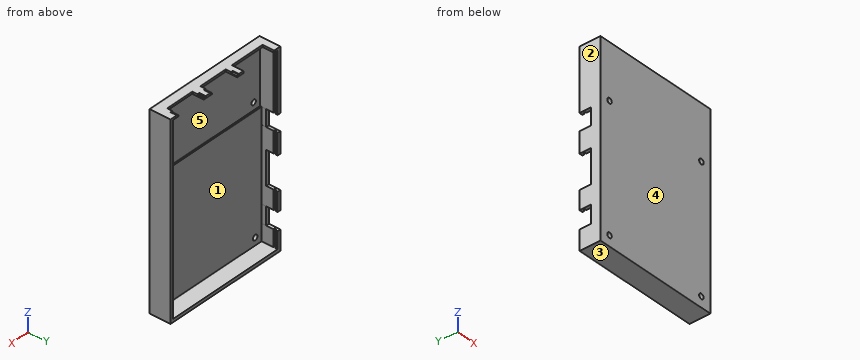
Autodesk Inventor part; units mm, degrees
ref_plane "YZ Plane" through (0, 0, 0) normal (1, 0, 0) x (0, 1, 0)
ref_plane "XZ Plane" through (0, 0, 0) normal (0, 1, 0) x (-1, 0, 0)
ref_plane "XY Plane" through (0, 0, 0) normal (0, 0, 1) x (1, 0, 0)
sketch "Sketch1" plane through (0, 0, 0) normal (0, 1, 0) x (-1, 0, 0)
  line L0 (89.3441, 14.7035) -> (28.3441, 14.7035)
  line L1 (28.3441, 14.7035) -> (28.3441, -75.7965)
  line L2 (28.3441, -75.7965) -> (89.3441, -75.7965)
  line L3 (89.3441, -75.7965) -> (89.3441, 14.7035)
  point P0 (0, 0)
  dimension "d0" = 90.5
  dimension "d1" = 61
extrude "Extrusion1" add sketch "Sketch1" along normal blind 1.5
sketch "Sketch2" plane through (0, 1.5, 0) normal (0, 1, 0) x (1, 0, 0)
  line L0 (-87.8441, -13.7035) -> (-29.8441, -13.7035)
  line L1 (-29.8441, -13.7035) -> (-29.8441, 74.2965)
  line L2 (-29.8441, 74.2965) -> (-87.8441, 74.2965)
  line L3 (-87.8441, 74.2965) -> (-87.8441, -13.7035)
  line L4 (-28.3441, 75.7965) -> (-89.3441, 75.7965)
  line L5 (-89.3441, -14.7035) -> (-28.3441, -14.7035)
  line L6 (-28.3441, -14.7035) -> (-28.3441, 75.7965)
  line L7 (-89.3441, 75.7965) -> (-89.3441, -14.7035)
  point P0 (0, 0)
  dimension "d4" = 1.5
  dimension "d5" = 1
  dimension "d6" = 1.5
  dimension "d7" = 1.5
extrude "Extrusion2" add sketch "Sketch2" along normal blind 8.5
sketch "Sketch3" plane through (-89.3441, 0, 14.7035) normal (0, 0, 1) x (1, 0, 0)
  line L0 (61, 0) -> (61, 10)
  line L1 (0, 0) -> (0, 10)
  line L2 (59.5, 1.5) -> (59.5, 10)
  line L3 (1.5, 1.5) -> (1.5, 10)
  line L4 (0, 0) -> (61, 0)
  line L5 (1.5, 1.5) -> (59.5, 1.5)
  line L6 (0, 10) -> (61, 10)
  line L7 (42.5, 10) -> (56.5, 10)
  line L8 (56.5, 10) -> (56.5, 1.5)
  line L9 (56.5, 1.5) -> (42.5, 1.5)
  line L10 (42.5, 1.5) -> (42.5, 10)
  line L11 (24, 10) -> (38, 10)
  line L12 (38, 10) -> (38, 1.5)
  line L13 (38, 1.5) -> (24, 1.5)
  line L14 (24, 1.5) -> (24, 10)
  line L15 (3.5, 10) -> (20.5, 10)
  line L16 (20.5, 10) -> (20.5, 1.5)
  line L17 (20.5, 1.5) -> (3.5, 1.5)
  line L18 (3.5, 1.5) -> (3.5, 10)
  point P0 (89.3441, 0)
  dimension "d10" = 61
  dimension "d11" = 58
  dimension "d12" = 1.5
  dimension "d13" = 10
  dimension "d14" = 3
  dimension "d15" = 14
  dimension "d16" = 14
  dimension "d17" = 4.5
  dimension "d18" = 3.5
  dimension "d19" = 17
  dimension "d20" = 2
extrude "Extrusion3" cut sketch "Sketch3" against normal blind 2 contours L8 L5 L10 L6 | L6 L16 L5 L18 | L12 L5 L14 L6
sketch "Sketch4" plane through (-89.3441, 0, -75.7965) normal (-1, 0, 0) x (0, 0, 1)
  line L0 (90.5, 0) -> (90.5, 10)
  line L1 (0, 0) -> (0, 10)
  line L2 (89.5, 1.5) -> (89.5, 10)
  line L3 (1.5, 1.5) -> (1.5, 10)
  line L4 (0, 0) -> (90.5, 0)
  line L5 (1.5, 1.5) -> (89.5, 1.5)
  line L6 (0, 10) -> (90.5, 10)
  line L7 (61, 10) -> (53, 10)
  line L8 (53, 10) -> (53, 1.5)
  line L9 (53, 1.5) -> (61, 1.5)
  line L10 (61, 1.5) -> (61, 10)
  line L11 (89.5, 10) -> (1.5, 10)
  line L12 (89.5, 1.5) -> (1.5, 1.5)
  line L13 (27, 10) -> (43, 10)
  line L14 (43, 10) -> (43, 1.5)
  line L15 (43, 1.5) -> (27, 1.5)
  line L16 (27, 1.5) -> (27, 10)
  line L17 (9.5, 10) -> (18, 10)
  line L18 (18, 10) -> (18, 1.5)
  line L19 (18, 1.5) -> (9.5, 1.5)
  line L20 (9.5, 1.5) -> (9.5, 10)
  point P0 (75.7965, 0)
  dimension "d23" = 90.5
  dimension "d24" = 88
  dimension "d25" = 1.5
  dimension "d26" = 10
  dimension "d27" = 28.5
  dimension "d28" = 8
  dimension "d29" = 10
  dimension "d30" = 16
  dimension "d31" = 9
  dimension "d32" = 8.5
  dimension "d33" = 8
extrude "Extrusion4" cut sketch "Sketch4" against normal blind 2 contours L10 L5 L8 L6 | L6 L18 L5 L20 | L14 L5 L16 L6
sketch "Sketch5" plane through (0, 10, 0) normal (0, 1, 0) x (1, 0, 0)
  line L0 (-29.8441, -13.7035) -> (-32.8441, -13.7035)
  line L1 (-32.8441, -14.7035) -> (-28.3441, -14.7035)
  line L2 (-28.3441, -14.7035) -> (-28.3441, 75.7965)
  line L3 (-32.8441, -13.7035) -> (-32.8441, -14.7035)
  line L4 (-32.8441, -14.7035) -> (-32.8441, -13.7035)
  line L5 (-89.3441, -14.7035) -> (-28.3441, -14.7035)
  line L6 (-32.8441, -14.2035) -> (-31.8441, -14.2035)
  line L7 (-31.8441, -14.2035) -> (-31.8441, -14.7035)
  line L8 (-31.8441, -14.7035) -> (-32.8441, -14.7035)
  line L9 (-32.8441, -14.7035) -> (-32.8441, -14.2035)
  point P0 (0, 0)
  dimension "d36" = 1
  dimension "d37" = 4.5
  dimension "d38" = 0.5
  dimension "d39" = 1
extrude "Extrusion5" cut sketch "Sketch5" against normal blind 3
sketch "Sketch6" plane through (0, 10, 0) normal (0, 1, 0) x (1, 0, 0)
  line L0 (-51.3441, -14.7035) -> (-46.8441, -14.7035)
  line L1 (-46.8441, -13.7035) -> (-51.3441, -13.7035)
  line L2 (-46.8441, -14.7035) -> (-46.8441, -13.7035)
  line L3 (-51.3441, -14.7035) -> (-51.3441, -13.7035)
  line L4 (-46.8441, -14.2035) -> (-47.8441, -14.2035)
  line L5 (-47.8441, -14.2035) -> (-47.8441, -14.7035)
  line L6 (-47.8441, -14.7035) -> (-46.8441, -14.7035)
  line L7 (-46.8441, -14.7035) -> (-46.8441, -14.2035)
  point P0 (0, 0)
  dimension "d42" = 1
  dimension "d43" = 4.5
  dimension "d44" = 0.5
  dimension "d45" = 1
extrude "Extrusion6" cut sketch "Sketch6" against normal blind 3 contours L5 L4 L2 L0
sketch "Sketch7" plane through (0, 10, 0) normal (0, 1, 0) x (1, 0, 0)
  line L0 (-46.8441, -13.7035) -> (-51.3441, -13.7035)
  line L1 (-51.3441, -14.7035) -> (-47.8441, -14.7035)
  line L2 (-46.8441, -14.2035) -> (-46.8441, -13.7035)
  line L3 (-51.3441, -13.7035) -> (-51.3441, -14.7035)
  line L4 (-46.8441, -14.7035) -> (-47.8441, -14.7035)
  line L5 (-47.8441, -14.2035) -> (-46.8441, -14.2035)
  line L6 (-51.3441, -14.2035) -> (-50.3441, -14.2035)
  line L7 (-50.3441, -14.2035) -> (-50.3441, -14.7035)
  line L8 (-50.3441, -14.7035) -> (-51.3441, -14.7035)
  line L9 (-51.3441, -14.7035) -> (-51.3441, -14.2035)
  point P0 (0, 0)
  dimension "d48" = 1
  dimension "d49" = 4.5
  dimension "d50" = 0.5
  dimension "d51" = 0.5
  dimension "d52" = 1
extrude "Extrusion7" cut sketch "Sketch7" against normal blind 3
sketch "Sketch8" plane through (0, 10, 0) normal (0, 1, 0) x (1, 0, 0)
  line L0 (-65.3441, -13.7035) -> (-68.8441, -13.7035)
  line L1 (-68.8441, -14.7035) -> (-65.3441, -14.7035)
  line L2 (-68.8441, -13.7035) -> (-68.8441, -14.7035)
  line L3 (-65.3441, -14.7035) -> (-65.3441, -13.7035)
  line L4 (-65.3441, -14.7035) -> (-65.3441, -13.7035)
  line L5 (-65.3441, -14.2035) -> (-66.3441, -14.2035)
  line L6 (-66.3441, -14.2035) -> (-66.3441, -14.7035)
  line L7 (-66.3441, -14.7035) -> (-65.3441, -14.7035)
  line L8 (-65.3441, -14.7035) -> (-65.3441, -14.2035)
  point P0 (0, 0)
  dimension "d55" = 1
  dimension "d56" = 3.5
  dimension "d57" = 1
  dimension "d58" = 0.5
extrude "Extrusion8" cut sketch "Sketch8" against normal blind 3 contours L3 L1 L6 L5
sketch "Sketch9" plane through (-29.8441, 1.5, -74.2965) normal (-1, 0, 0) x (0, 0, 1)
  line L0 (0, 0) -> (0, 8.5)
  line L1 (0, 7.5) -> (88.9462, 7.5)
  line L2 (88.9462, 7.5) -> (88.9462, 6.5)
  line L3 (88.9462, 6.5) -> (0, 6.5)
  line L4 (0, 6.5) -> (0, 7.5)
  line L5 (0, 8.5) -> (88, 8.5)
  point P0 (74.2965, -1.5)
  dimension "d61" = 1
  dimension "d62" = 88.9462
  dimension "d63" = 1
extrude "Extrusion9" cut sketch "Sketch9" against normal blind 0.5
sketch "Sketch10" plane through (-87.8441, 1.5, 13.7035) normal (1, 0, 0) x (0, 0, -1)
  line L0 (28.5, 0) -> (28.5, 8.5)
  line L1 (0, 7.5) -> (28.5, 7.5)
  line L2 (28.5, 7.5) -> (28.5, 6.5)
  line L3 (28.5, 6.5) -> (0, 6.5)
  line L4 (0, 6.5) -> (0, 7.5)
  line L5 (0, 8.5) -> (28.5, 8.5)
  point P0 (13.7035, -1.5)
  dimension "d66" = 28.5
  dimension "d67" = 1
  dimension "d68" = 1
extrude "Extrusion10" cut sketch "Sketch10" against normal blind 0.5
sketch "Sketch11" plane through (-87.8441, 1.5, -22.7965) normal (1, 0, 0) x (0, 0, -1)
  line L0 (0, 8.5) -> (0, 0)
  line L1 (10, 0) -> (10, 8.5)
  line L2 (0, 7.5) -> (10, 7.5)
  line L3 (10, 7.5) -> (10, 6.5)
  line L4 (10, 6.5) -> (0, 6.5)
  line L5 (0, 6.5) -> (0, 7.5)
  line L6 (0, 8.5) -> (10, 8.5)
  point P0 (-22.7965, -1.5)
  dimension "d71" = 10
  dimension "d72" = 1
  dimension "d73" = 1
extrude "Extrusion11" cut sketch "Sketch11" against normal blind 0.5 contours L2 L1 L4 L0
sketch "Sketch12" plane through (-87.8441, 1.5, -48.7965) normal (1, 0, 0) x (0, 0, -1)
  line L0 (0, 8.5) -> (0, 0)
  line L1 (9, 0) -> (9, 8.5)
  line L2 (0, 7.5) -> (9, 7.5)
  line L3 (9, 7.5) -> (9, 6.5)
  line L4 (9, 6.5) -> (0, 6.5)
  line L5 (0, 6.5) -> (0, 7.5)
  line L6 (0, 8.5) -> (9, 8.5)
  point P0 (-48.7965, -1.5)
  dimension "d76" = 1
  dimension "d77" = 1
extrude "Extrusion12" cut sketch "Sketch12" against normal blind 0.5 contours L2 L1 L4 L0
sketch "Sketch13" plane through (-87.8441, 1.5, -74.2965) normal (1, 0, 0) x (0, 0, -1)
  line L0 (0, 0) -> (0, 8.5)
  line L1 (-8, 8.5) -> (-8, 0)
  line L2 (0, 7.5) -> (-8, 7.5)
  line L3 (-8, 7.5) -> (-8, 6.5)
  line L4 (-8, 6.5) -> (0, 6.5)
  line L5 (0, 6.5) -> (0, 7.5)
  line L6 (-8, 8.5) -> (0, 8.5)
  point P0 (-74.2965, -1.5)
  dimension "d80" = 1
  dimension "d81" = 1
extrude "Extrusion13" cut sketch "Sketch13" against normal blind 0.5 contours L4 L1 L2 L0
sketch "Sketch16" plane through (0, 1.5, 0) normal (0, 1, 0) x (1, 0, 0)
  line L0 (-87.8539, 14.7789) -> (-29.8441, 14.7789)
  line L1 (-29.8441, 14.7789) -> (-29.8441, 74.2965)
  line L2 (-29.8441, 74.2965) -> (-87.8539, 74.2965)
  line L3 (-87.8539, 74.2965) -> (-87.8539, 14.7789)
  line L4 (-89.3441, 22.7965) -> (-87.8539, 22.7965)
  line L5 (-87.8539, 22.7965) -> (-87.8539, 14.7789)
  line L6 (-87.8539, 14.7789) -> (-89.3441, 14.7789)
  line L7 (-89.3441, 14.7789) -> (-89.3441, 22.7965)
  line L8 (-89.3441, 48.7965) -> (-87.8441, 48.7965)
  line L9 (-87.8441, 48.7965) -> (-87.8441, 32.7965)
  line L10 (-87.8441, 32.7965) -> (-89.3441, 32.7965)
  line L11 (-89.3441, 32.7965) -> (-89.3441, 48.7965)
  line L12 (-89.3441, 66.2965) -> (-87.8539, 66.2965)
  line L13 (-87.8539, 66.2965) -> (-87.8539, 57.7072)
  line L14 (-87.8539, 57.7072) -> (-89.3441, 57.7072)
  line L15 (-89.3441, 57.7072) -> (-89.3441, 66.2965)
  line L16 (-89.3441, 66.2965) -> (-87.8539, 66.2965)
  line L17 (-87.8539, 66.2965) -> (-87.8539, 57.7072)
  line L18 (-87.8539, 57.7072) -> (-89.3441, 57.7072)
  line L19 (-89.3441, 57.7072) -> (-89.3441, 66.2965)
  line L20 (-85.8441, -13.7035) -> (-68.8441, -13.7035)
  line L21 (-68.8441, -13.7035) -> (-68.8441, -14.7035)
  line L22 (-68.8441, -14.7035) -> (-85.8441, -14.7035)
  line L23 (-85.8441, -14.7035) -> (-85.8441, -13.7035)
  line L24 (-65.3441, -13.7035) -> (-51.3441, -13.7035)
  line L25 (-51.3441, -13.7035) -> (-51.3441, -14.7035)
  line L26 (-51.3441, -14.7035) -> (-65.3441, -14.7035)
  line L27 (-65.3441, -14.7035) -> (-65.3441, -13.7035)
  line L28 (-46.8441, -13.7035) -> (-32.8441, -13.7035)
  line L29 (-32.8441, -13.7035) -> (-32.8441, -14.7035)
  line L30 (-32.8441, -14.7035) -> (-46.8441, -14.7035)
  line L31 (-46.8441, -14.7035) -> (-46.8441, -13.7035)
  point P0 (0, 0)
extrude "Extrusion16" add sketch "Sketch16" along normal blind 3 contours L6 L7 L4 L3 | L10 L11 L8 L3 | L3 L8 L9 L10 | L3 L14 L15 L12 | L20 L21 L22 L23 | L24 L25 L26 L27 | L28 L29 L30 L31
sketch "Sketch17" plane through (0, 1.5, 0) normal (0, 1, 0) x (1, 0, 0)
  line L0 (-87.8539, 14.7965) -> (-29.8441, 14.7965)
  line L1 (-29.8441, 14.7965) -> (-29.8441, 74.2965)
  line L2 (-29.8441, 74.2965) -> (-87.8539, 74.2965)
  line L3 (-87.8539, 74.2965) -> (-87.8539, 14.7965)
  point P0 (0, 0)
extrude "Extrusion17" add sketch "Sketch17" along normal blind 0.75
hole "Hole1" at (-84.3441, 1.5, -11.2965) direction (0, -1, 0) diameter 2.5 end through all
hole "Hole2" at (-33.3441, 1.5, -11.1445) direction (0, -1, 0) diameter 2.5 end through all
hole "Hole3" at (-84.3441, 2.25, -70.7965) direction (0, -1, 0) diameter 2.5 end through all
hole "Hole4" at (-33.3441, 2.25, -70.7965) direction (0, -1, 0) diameter 2.5 end through all
properties part number "raspi_enclosure"
Geometry check sheet. Reference: the model listing, model coordinates, mm. Face numbers are marked on the shaded views. A direction names the side the tool comes from. Round coordinates to 2 decimals unless told otherwise and drop trailing zeros. Loops run counter-clockwise (first coordinate to the right, second up) from the corner with the lowest first, then second, coordinate; pieces in that order, holes last.
Item 1: Cross-section at C-C on z = -5.5. Record the boundary of the cut face in (x, y).
Item 2: Mould release check, pull along Z, two halves, no side actions. Record for the marked faces 1, 2 and 3: pulls with the +Z half, pulls with the -Z half, needs draft (parallel to the pull), parting line crosses it, or undercut.
Item 3: Gauge pin test, flat ends, axial feed: pin 1 (3 mm diameter, centred on x = -55, z = -16.5, fed in from +Y); pin 2 (6 mm diameter, centred on x = -61.5, y = 8, fed in from +Z); pin 3 (6 mm diameter, centred on x = -53, z = -5.5, fed in from +Y). Record the tip position at first contact, or that the pin passes through.
Item 4: Cross-section at B-B on x = -75.5. Record the boundary of the cut face in (y, z), then the cut area to 3 significant figures.
Item 5: Access from +Z, -Z, +X, -X, +Y, -Y to the whole of each face (thin tool, end or side, straight path). Record for the marked faces 4 and 5.
Item 6: Cross-section at A-A on z = -54. Record the boundary of the cut face in (x, y).
Item 7: Thickness scan on line 1 (X direction, y = 2.5, z = 2.5); line 2 (Z direction, x = -76, y = 2); line 3 (X direction, y = 3, z = -60.5). Record the ranges inside material, lowest first.
Answer sheet:
1. outline: (-89.34, 0) - (-28.34, 0) - (-28.34, 10) - (-29.84, 10) - (-29.84, 9) - (-29.34, 9) - (-29.34, 8) - (-29.84, 8) - (-29.84, 1.5) - (-87.84, 1.5) - (-87.84, 8) - (-88.34, 8) - (-88.34, 9) - (-87.84, 9) - (-87.84, 10) - (-89.34, 10) - close
2. face 1: undercut
2. face 2: needs draft
2. face 3: pulls with the -Z half
3. pin 1: stops at y = 2.25
3. pin 2: stops at z = -74.3
3. pin 3: stops at y = 1.5
4. outline: (0, -75.8) - (10, -75.8) - (10, -74.3) - (2.25, -74.3) - (2.25, -14.8) - (1.5, -14.8) - (1.5, 13.7) - (4.5, 13.7) - (4.5, 14.7) - (0, 14.7) - close
4. area: 196 mm2
5. face 4: +Z, -Z, +X, -X, -Y
5. face 5: +Y
6. outline: (-89.34, 0) - (-28.34, 0) - (-28.34, 10) - (-29.84, 10) - (-29.84, 9) - (-29.34, 9) - (-29.34, 8) - (-29.84, 8) - (-29.84, 2.25) - (-87.84, 2.25) - (-87.84, 8) - (-88.34, 8) - (-88.34, 9) - (-87.84, 9) - (-87.84, 10) - (-89.34, 10) - close
7. line 1: x = -89.34 to -87.84, -29.84 to -28.34
7. line 2: z = -75.8 to -14.8, 13.7 to 14.7
7. line 3: x = -89.34 to -87.85, -29.84 to -28.34
